Could you check a few things on this model? Use its own coordinates, in mm. Coordinates: 2 decimals unless noted, no trailing zeros. Loops run counter-clockwise (first coordinate to the right, second up) from the corner with the lowest first, then second, coordinate; pieces in that order, holes last. Notation, with made-up numbers: (-6.75, 78.25) - (6.25, 78.25) arc R15 cw to (6.25, 90.25) - close; hole circle Ø8 at (57.5, 77). An arc over 180 degrees is marked (long way). One line per item, written item: value. Start each with the question number.
(1) If I drill on line 1 along Z through (x, y) = (8, -2.4); line 2 along X through (y, z) = (-1.9, -1); line 3 along Y through (x, z) = (41, 5.75) (3 decimals), over which ranges is the centre line in solid material (lowest first)? Write a range as from..to.
(2) If we section it at C-C on y = -1.2: Write out the boundary of the cut face in (x, z).
(3) If we section it at A-A on y = -3.9: Write out the boundary of the cut face in (x, z), then the cut area to 3 significant figures.
(4) I'm going to push flat-ended pins straight in: P1, Ø1, axis at x = 44, y = -4, coming from the +Z side; P2, Ø1, axis at x = 44, y = -4, coming from the -Z side. Where does each tip first touch, or does it pass through?
```python
from build123d import *

# Parameters (mm, degrees)
F0_W     = 12.7
F0_H     = 12.7
F1_DEPTH = 4.7625
F2_W     = 38.1
F2_H     = 12.7
F2_W_2   = 34.925
F2_H_2   = 9.525
F3_DEPTH = 3.175
F4_W     = 1.5875
F4_H     = 0.635
F5_DEPTH = 1.5875
F6_SIZE  = 0.31749


# Not quite as in the source:
# - a fillet or chamfer is up to 0.001 mm smaller than in the source, because OpenCascade refuses the exact size


with BuildPart() as f1:
    # F0 (on Front) → F1 (new body)
    with BuildSketch(Plane.XZ):
        Rectangle(F0_W, F0_H)
    extrude(amount=F1_DEPTH)

    # F2 (on Front) → F3 (join)
    with BuildSketch(Plane.XZ):
        with Locations((25.4, 0)):
            Rectangle(F2_W, F2_H)
        with Locations((25.4, 0)):
            Rectangle(F2_W_2, F2_H_2, mode=Mode.SUBTRACT)
    extrude(amount=F3_DEPTH)

    # F4 (on face) → F5 (join)
    with BuildSketch(Plane.XZ.offset(3.175)):
        with Locations((43.65625, 0)):
            Rectangle(F4_W, F4_H)
    extrude(amount=F5_DEPTH)

    # F6 (size 0.3175 in the source; OpenCascade refuses exactly that, so slightly less here)
    f6_edges = [f1.edges().sort_by_distance(p)[0] for p in [
        (43.65625, -4.7625, 0.3175),
        (42.8625, -4.7625, 0),
        (43.65625, -4.7625, -0.3175),
        (44.45, -4.7625, 0),
    ]]
    chamfer(f6_edges, length=F6_SIZE)


solid = f1.part
```
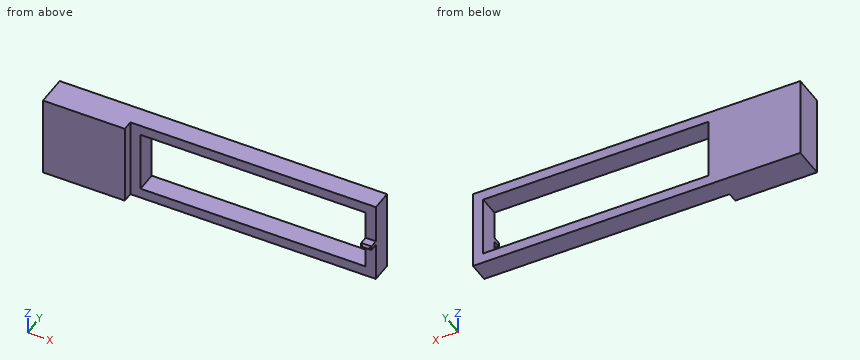
Values:
1. line 1: z = -6.35..-4.76, 4.76..6.35
1. line 2: x = -6.35..7.94, 42.86..44.45
1. line 3: y = -3.175..0
2. outline: (-6.35, -6.35) - (44.45, -6.35) - (44.45, 6.35) - (-6.35, 6.35) - close; hole (7.94, -4.76) - (42.86, -4.76) - (42.86, 4.76) - (7.94, 4.76) - close
3. outline: (-6.35, -6.35) - (6.35, -6.35) - (6.35, 6.35) - (-6.35, 6.35) - close; (42.86, -0.32) - (44.45, -0.32) - (44.45, 0.32) - (42.86, 0.32) - close
3. area: 162 mm2
4. P1: stops at z = 0.32
4. P2: stops at z = -0.32
